Could you check a few things on this model? Use its own coordinates, in mm. Coordinates: 2 decimals unless noted, no trailing zeros. Loops run counter-clockwise (first coordinate to the right, second up) from the corner with the lowest first, then second, coordinate; pieces in that order, holes last.
from build123d import *

# Parameters (mm, degrees)
SKETCH1_R           = 46
SKETCH1_R_2         = 36
BOSS_EXTRUDE1_DEPTH = 3
CHAMFER1_SIZE       = 2
SKETCH2_R           = 1.7
CUT_EXTRUDE1_DEPTH  = 66.122960621
CIRPATTERN1_COUNT   = 3
CHAMFER2_SIZE       = 1


with BuildPart() as part:
    # Sketch1 → Boss-Extrude1 (new body)
    with BuildSketch(Plane(origin=(0, 0, 0), x_dir=(1, 0, 0), z_dir=(0, 1, 0))):
        with Locations(Location((0, 0, 0), (0, 0, 270))):
            Circle(SKETCH1_R)
        with Locations(Location((0, 0, 0), (0, 0, 270))):
            Circle(SKETCH1_R_2, mode=Mode.SUBTRACT)
    extrude(amount=BOSS_EXTRUDE1_DEPTH)

    # Chamfer1
    chamfer1_edges = [part.edges().sort_by_distance(p)[0] for p in [
        (0, 3, -46),
    ]]
    chamfer(chamfer1_edges, length=CHAMFER1_SIZE)

    # Sketch2 → Cut-Extrude1 (cut, through all)
    with BuildSketch(Plane(origin=(0, 3, 0), x_dir=(1, 0, 0), z_dir=(0, 1, 0))):
        with Locations(Location((0, 39.251, 0), (0, 0, 270))):
            Circle(SKETCH2_R)
    cut_extrude1 = extrude(amount=-CUT_EXTRUDE1_DEPTH, mode=Mode.SUBTRACT)

    # CirPattern1: Cut-Extrude1 ×3 about axis
    cirpattern1_axis = Axis((0, 0, 0), (0, 1, 0))
    for i in range(1, CIRPATTERN1_COUNT):
        add(cut_extrude1.rotate(cirpattern1_axis, i * 360 / CIRPATTERN1_COUNT), mode=Mode.SUBTRACT)

    # Chamfer2
    chamfer2_edges = [part.edges().sort_by_distance(p)[0] for p in [
        (0, 3, -36),
    ]]
    chamfer(chamfer2_edges, length=CHAMFER2_SIZE)


solid = part.part
(1) For pin 1 (2 mm diameter, centred on x = 33.99, z = 19.63, fed in from -Y); pin 2 (12 mm diameter, centred on x = 9.5, z = 31.5, fed in from +Y), each with a flat end and sliding along its axis, tell me the tip position at first contact or that it passes through.
Answers:
pin 1: passes through
pin 2: stops at y = 3
(2) Imagine slicing it at D-D, the plane x = -34. State how many separate pieces and enclosed holes the cut face has, and give its area (3 significant figures).
Answers:
separate pieces: 3
enclosed holes: 0
area: 95.8 mm2
(3) Imagine slicing it at C-C, the plane y = 0.55. Write out the boundary of the cut face in (x, z).
Answers:
outline: circle Ø92 at (0, 0); hole circle Ø72 at (0, 0); hole circle Ø3.4 at (-33.99, 19.63); hole circle Ø3.4 at (0, -39.25); hole circle Ø3.4 at (33.99, 19.63)
(4) We'd pull the mould along X, two halves only. Please class faces 1 (the face through (-23.6, 0, -27.5)), 2 (the face through (10.81, 0.99, 34.34)), 3 (the face through (38.787, 0.493, 24.729)), 4 (the face through (35.14, 1.52, 18.37)): +X half, -X half, draft (parallel to the pull), parting line (faces both ways), or undercut.
Answers:
face 1: draft
face 2: undercut
face 3: parting line
face 4: undercut
(5) I need wall thicknesses on probe 1 along Z at (x, y) = (1.5, 2.3); probe 2 along X at (y, z) = (1, 0); probe 3 along X at (y, z) = (2.55, -9). Which ranges of each line are inside material? Lowest first, please.
Answers:
probe 1: z = -44.67 to -40.05, -38.45 to -36.27, 36.27 to 44.67
probe 2: x = -46 to -36, 36 to 46
probe 3: x = -43.53 to -35.42, 35.42 to 43.53
(6) Imagine slicing it at B-B, the plane z = 0. Write out the boundary of the cut face in (x, y), and give its area (3 significant figures).
Answers:
outline: (-46, 0) - (-36, 0) - (-36, 2) - (-37, 3) - (-44, 3) - (-46, 1) - close; (36, 0) - (46, 0) - (46, 1) - (44, 3) - (37, 3) - (36, 2) - close
area: 55.0 mm2
(7) Imagine slicing it at A-A, the plane x = 0. Write out the boundary of the cut face in (y, z), and give its area (3 significant figures).
Answers:
outline: (0, -46) - (1, -46) - (3, -44) - (3, -40.95) - (0, -40.95) - close; (0, -37.55) - (3, -37.55) - (3, -37) - (2, -36) - (0, -36) - close; (0, 36) - (2, 36) - (3, 37) - (3, 44) - (1, 46) - (0, 46) - close
area: 44.8 mm2
